Verification items for the finished model (mm, model axes). A direction names the side the tool comes from. Coordinates: 2 decimals unless noted, no trailing zeros. Order: outer loops, then holes, each group sorted by start corner. A loop starts at its lowest first (then second) coordinate and runs counter-clockwise, first axis right, second up.
Q1. Depth check by flat-ended pin: P1, Ø6, axis at x = 16, y = -26.5, coming from the +Z side; P2, Ø4, axis at y = -8, z = 7, coming from the +X side; P3, Ø8, axis at x = 16.5, z = 15.5, coming from the +Y side; P4, Ø8, axis at x = -8, z = 21, coming from the -Y side. Enter the tip coordinate at first touch or a pass-through.
Q2. Cross-section at B-B, the plane y = -28. Record the boundary of the cut face in (x, z), and give its area (3 significant figures).
Q3. Cross-section at C-C, the plane x = 6. Record the boundary of the cut face in (y, z).
Q4. Cross-section at A-A, the plane z = 16.5. Record the boundary of the cut face in (x, y) (3 decimals).
Q5. Thickness scan on line 1 (X direction, y = -24.5, z = 10.75); line 2 (X direction, y = 12, z = 14.25); line 3 (Y direction, x = -15.5, z = 22.75). Record the ranges inside material, lowest first.
Q6. Set-up check for faces 1 (the flat face through (0, -14, 0)), 2 (the flat face through (-12.793, -28, 13)), 3 (the flat face through (12.607, -28, 13)): record each of +Z, -Z, +X, -X, +Y, -Y from which the full face is reachable in a straight line by a thin tool's end or side.
from build123d import *

# Parameters (mm, degrees)
F1_DEPTH = 25.4


with BuildPart() as f1:
    # F0 (on Top) → F1 (new body)
    with BuildSketch(Plane.XY):
        with BuildLine():
            Line((12.607468, -38.099831), (12.607468, -18.30307))
            ThreePointArc((12.607468, -18.30307), (21.22188, 6.6017), (0, 22.225))
            ThreePointArc((0, 22.225), (-21.188114, 6.709281), (-12.792532, -18.174206))
            Line((-12.792532, -18.174206), (-12.792532, -38.099831))
            ThreePointArc((-12.792532, -38.099831), (-0.092532, -50.799831), (12.607468, -38.099831))
        make_face()
    extrude(amount=F1_DEPTH)


solid = f1.part
Check values:
1. P1: passes through
1. P2: stops at x = 21.4
1. P3: stops at y = 18.38
1. P4: stops at y = -50.18
2. outline: (-12.79, 0) - (12.61, 0) - (12.61, 25.4) - (-12.79, 25.4) - close
2. area: 645 mm2
3. outline: (-49.24, 0) - (21.4, 0) - (21.4, 25.4) - (-49.24, 25.4) - close
4. outline: (-12.793, -38.1) arc R12.7 ccw to (12.607, -38.1) - (12.607, -18.303) arc R22.225 ccw (long way) to (-12.793, -18.174) - close
5. line 1: x = -12.79 to 12.61
5. line 2: x = -18.71 to 18.71
5. line 3: y = -15.93 to 15.93
6. face 1: -Z, +X, -X, +Y, -Y
6. face 2: +Z, -Z, -X, -Y
6. face 3: +Z, -Z, +X, -Y
